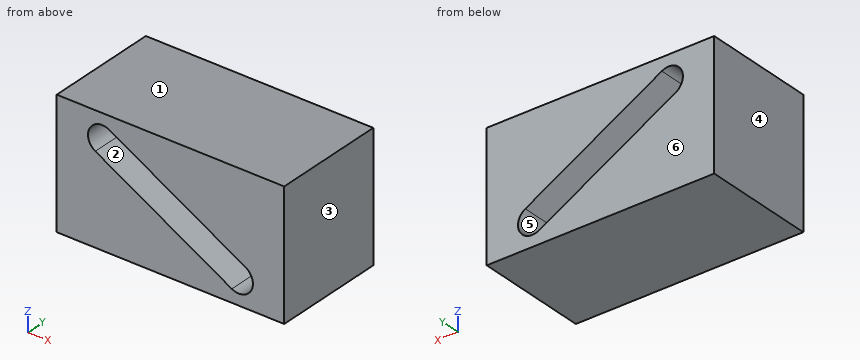
```python
from build123d import *

# Parameters (mm, degrees)
F0_W     = 18
F0_H     = 10
F1_DEPTH = 4.5


with BuildPart() as f1:
    # F0 (on Front) → F1 (new body, symmetric)
    with BuildSketch(Plane.XZ):
        Rectangle(F0_W, F0_H)
        with BuildLine():
            ThreePointArc((-5.946348, 2.016573), (-6.383427, 3.546348), (-4.853652, 3.983427))
            Line((-4.853652, 3.983427), (5.946348, -2.016573))
            ThreePointArc((5.946348, -2.016573), (6.383427, -3.546348), (4.853652, -3.983427))
            Line((4.853652, -3.983427), (-5.946348, 2.016573))
        make_face(mode=Mode.SUBTRACT)
    extrude(amount=F1_DEPTH, both=True)


solid = f1.part
```
Verification items for the finished model (mm, model axes). Face numbers are marked on the shaded views. A direction names the side the tool comes from. Round coordinates to 2 decimals unless told otherwise and drop trailing zeros. Write each loop counter-clockwise with the first axis right and the second up, starting at its lowest first coordinate (ties: lowest second). Pieces come first, ordered by that corner, then holes. Notation, with made-up numbers: (41.5, 2.5) - (61.5, 2.5) arc R18 ccw to (61.5, 6.5) - close; hole circle Ø8 at (-21, -18.75). An arc over 180 degrees is marked (long way). Answer as a JSON object with one key per item and string values. Group by question number.
Q1. Mould release check, pull along X, two halves, no side actions. Record for the marked faces 3, 4, 5 and 6: released by +X, released by -X, zero draft, split by the parting line, or undercut.
Q2. Tool access check on the marked faces 1 and 2. Record the directions out of +Z, -Z, +X, -X, +Y, -Y that give a thin tool (end or side, any length) a straight path to the whole face; none if there is none.
Q3. Thickness scan on line 1 (X direction, y = -2.75, z = 3) (3 decimals); line 2 (X direction, y = 2, z = 2); line 3 (Z direction, x = 6, y = -2). Record the ranges inside material, lowest first.
Q4. Section check B-B, the plane y = -0.25. Enter the section's corners in (x, z) (3 decimals), plus the area to 3 significant figures.
Q5. Section check A-A, the plane x = 4.5. Enter the section's corners in (y, z), plus the area to 3 significant figures.
Q6. Section check C-C, the plane z = -1.25. Enter the section's corners in (x, y).
Found:
{
 "1": {"face 3": "released by +X", "face 4": "released by -X", "face 5": "undercut", "face 6": "zero draft"},
 "2": {"face 1": "+Z, +X, -X, +Y, -Y", "face 2": "+Y, -Y"},
 "3": {"line 1": "x = -9 to -6.525, -3.083 to 9", "line 2": "x = -9 to -5.92, -1.28 to 9", "line 3": "z = -5 to -3.95, -2.05 to 5"},
 "4": {"outline": "(-9, -5) - (9, -5) - (9, 5) - (-9, 5) - close; hole (-5.946, 2.017) - (4.854, -3.983) arc R1.125 ccw to (5.946, -2.017) - (-4.854, 3.983) arc R1.125 ccw to start", "area": "148 mm^2"},
 "5": {"outline": "(-4.5, -5) - (4.5, -5) - (4.5, -3.79) - (-4.5, -3.79) - close; (-4.5, -1.21) - (4.5, -1.21) - (4.5, 5) - (-4.5, 5) - close", "area": "66.8 mm^2"},
 "6": {"outline": "(-9, -4.5) - (-0.07, -4.5) - (-0.07, 4.5) - (-9, 4.5) - close; (4.57, -4.5) - (9, -4.5) - (9, 4.5) - (4.57, 4.5) - close"}
}
